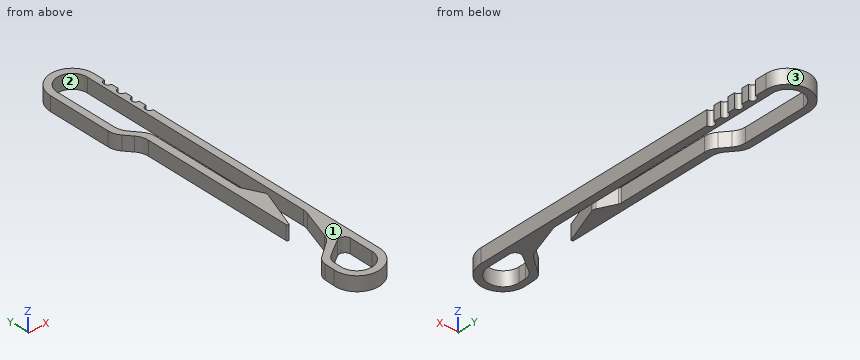
```python
from build123d import *

# Parameters (mm, degrees)
F1_DEPTH = 2.5
F2_R     = 1
F3_R     = 0.2
F4_R     = 1
F5_R     = 3
F6_R     = 3
F7_R     = 3
F8_R     = 3
F9_R     = 2
F10_R    = 2
F11_R    = 3
F12_R    = 1


# Not quite as in the source:
# - ends of sketch curves that miss each other by under 0.0002 mm in the source are joined


with BuildPart() as f1:
    # F0 (on Top) → F1 (new body)
    with BuildSketch(Plane.XY):
        with BuildLine():
            Line((-3.7337125044, -24.7166411829), (-3.8395490403, -27.4549634883))
            ThreePointArc((-3.8395490403, -27.4549634883), (-0.0393100387, -31.4820484538), (3.9136249429, -27.6047381979))
            Line((3.9136249429, -27.6047381979), (3.9136249429, 15.7631997109))
            ThreePointArc((3.9136249429, 15.7631997109), (3.2136249429, 16.4631997109), (3.9136249429, 17.1631997109))
            Line((3.9136249429, 17.1631997109), (3.9136249429, 18.4257015441))
            ThreePointArc((3.9136249429, 18.4257015441), (3.2136249429, 19.1257015441), (3.9136249429, 19.8257015441))
            Line((3.9136249429, 19.8257015441), (3.9136249429, 21.0882033773))
            ThreePointArc((3.9136249429, 21.0882033773), (3.2136249429, 21.7882033773), (3.9136249429, 22.4882033773))
            Line((3.9136249429, 22.4882033773), (3.9136249429, 23.7507052105))
            ThreePointArc((3.9136249429, 23.7507052105), (3.2136249429, 24.4507052105), (3.9136249429, 25.1507052105))
            Line((3.9136249429, 25.1507052105), (3.9136249429, 27.1132070437))
            ThreePointArc((3.9136249429, 27.1132070437), (0.1053655494, 30.9191937737), (-3.7028938442, 27.1132070437))
            Line((-3.7028938442, 27.1132070437), (-3.7101279046, 14.9948472524))
            Line((-3.7101279046, 14.9948472524), (-1.3026787113, 12.0476867709))
            Line((-1.3026787113, 12.0476867709), (-1.3526145996, -16.6168491978))
            Line((-1.3526145996, -16.6168491978), (1.6919830966, -8.5560908617))
            Line((1.6919830966, -8.5560908617), (-0.0073911714, -5.1353744853))
            Line((-0.0073911714, -5.1353744853), (-0.0073911714, 12.04390363))
            Line((-0.0073911714, 12.04390363), (-2.5009698886, 15.147203732))
            Line((-2.5009698886, 15.147203732), (-2.5009698886, 27.3470994339))
            ThreePointArc((-2.5009698886, 27.3470994339), (0.2224335348, 29.7253272746), (2.7223778727, 27.1132070292))
            Line((2.7223778727, 27.1132070292), (2.7223883904, 27.1109336758))
            Line((2.7223883904, 27.1109336758), (2.6088146402, -14.972403604))
            Line((2.6088146402, -14.972403604), (0.3495425781, -21.5565683108))
            Line((0.3495425781, -21.5565683108), (-3.7337125044, -24.7166411829))
        make_face()
        with BuildLine():
            ThreePointArc((2.6714254586, -27.6047381979), (-0.0471437397, -30.2812376007), (-2.7139096259, -27.5531197061))
            Line((-2.7139096259, -27.5531197061), (-2.6834930082, -25.2417523976))
            Line((-2.6834930082, -25.2417523976), (2.7000635964, -21.5408525771))
            Line((2.7000635964, -21.5408525771), (2.6714254586, -27.6047381979))
        make_face(mode=Mode.SUBTRACT)
    extrude(amount=F1_DEPTH)

    # F2
    f2_edges = [f1.edges().sort_by_distance(p)[0] for p in [
        (2.700064, -21.540853, 1.25),
    ]]
    fillet(f2_edges, radius=F2_R)

    # F3
    f3_edges = [f1.edges().sort_by_distance(p)[0] for p in [
        (-1.352615, -16.616849, 1.25),
    ]]
    fillet(f3_edges, radius=F3_R)

    # F4
    f4_edges = [f1.edges().sort_by_distance(p)[0] for p in [
        (1.691983, -8.556091, 1.25),
    ]]
    fillet(f4_edges, radius=F4_R)

    # F5
    f5_edges = [f1.edges().sort_by_distance(p)[0] for p in [
        (-2.50097, 15.147204, 1.25),
    ]]
    fillet(f5_edges, radius=F5_R)

    # F6
    f6_edges = [f1.edges().sort_by_distance(p)[0] for p in [
        (-3.710128, 14.994847, 1.25),
    ]]
    fillet(f6_edges, radius=F6_R)

    # F7
    f7_edges = [f1.edges().sort_by_distance(p)[0] for p in [
        (-1.302679, 12.047687, 1.25),
    ]]
    fillet(f7_edges, radius=F7_R)

    # F8
    f8_edges = [f1.edges().sort_by_distance(p)[0] for p in [
        (-0.007391, 12.043904, 1.25),
    ]]
    fillet(f8_edges, radius=F8_R)

    # F9
    f9_edges = [f1.edges().sort_by_distance(p)[0] for p in [
        (-3.733713, -24.716641, 1.25),
    ]]
    fillet(f9_edges, radius=F9_R)

    # F10
    f10_edges = [f1.edges().sort_by_distance(p)[0] for p in [
        (-2.683493, -25.241752, 1.25),
    ]]
    fillet(f10_edges, radius=F10_R)

    # F11
    f11_edges = [f1.edges().sort_by_distance(p)[0] for p in [
        (0.349543, -21.556568, 1.25),
        (2.608815, -14.972404, 1.25),
    ]]
    fillet(f11_edges, radius=F11_R)

    # F12
    f12_edges = [f1.edges().sort_by_distance(p)[0] for p in [
        (-0.007391, -5.135374, 1.25),
    ]]
    fillet(f12_edges, radius=F12_R)


solid = f1.part
```
For this review, take the finished solid that the model builds, in its own axes (mm). Face numbers are marked on the shaded views. Coordinates: 2 decimals unless noted, no trailing zeros. Order: outer loops, then holes, each group sorted by start corner. A loop starts at its lowest first (then second) coordinate and runs counter-clockwise, first axis right, second up. Notation, with made-up numbers: (10, 85) -> (17, 85) arc R13 ccw to (17, 102) -> close; hole circle Ø5 at (17.5, 33). An arc over 180 degrees is marked (long way). Use CSV: the item, a comma, the result in double quotes. Start each with the question number.
Item 1: Wall thickness on probe 1 along X at (y, z) = (27, 1.2); probe 2 along X at (y, z) = (-13, 1.65); probe 3 along Y at (x, z) = (-1.25, 0.95): over which ranges is each line inside the solid? List them lowest first.
Item 2: We need section B-B, the plane y = 24.5. Give the boundary of the cut face in (x, z), then the cut area to 3 significant figures.
Item 3: Draft analysis for pull direction Y (two halves, no side actions). For the marked faces 1, 2 and 3, state which applies: pulls with the +Y half, pulls with the -Y half, needs draft (parallel to the pull), parting line crosses it, or undercut.
Item 4: Insertion check: pin 1 (1.5 mm diameter, centred on x = -2, z = 1.5, fed in from -Y). The pin has a flat end and moves straight along its axis. Give the tip position at first contact, or say it passes through.
Item 5: We need section A-A, the plane y = 9.5. Give the boundary of the cut face in (x, z), then the cut area to 3 significant figures.
Derived:
1,probe 1,"x = -3.7 to -2.5, 2.72 to 3.91"
1,probe 2,"x = -1.35 to 0.01, 2.61 to 3.91"
1,probe 3,"y = -31.26 to -29.98, -24.26 to -22.79, -15.69 to 13.59, 29.35 to 30.67"
2,outline,"(-3.7, 0) -> (-2.5, 0) -> (-2.5, 2.5) -> (-3.7, 2.5) -> close; (2.72, 0) -> (3.22, 0) -> (3.22, 2.5) -> (2.72, 2.5) -> close"
2,area,"4.26 mm^2"
3,face 1,"needs draft"
3,face 2,"undercut"
3,face 3,"pulls with the +Y half"
4,pin 1,"stops at y = -31.26"
5,outline,"(-1.31, 0) -> (-0.01, 0) -> (-0.01, 2.5) -> (-1.31, 2.5) -> close; (2.67, 0) -> (3.91, 0) -> (3.91, 2.5) -> (2.67, 2.5) -> close"
5,area,"6.35 mm^2"
